CAD build for the part. Positions are in the model's coordinates, mm. Face numbers are marked on the shaded views. Round coordinates to 2 decimals unless told otherwise and drop trailing zeros. Order: outer loops, then holes, each group sorted by start corner. A loop starts at its lowest first (then second) coordinate and runs counter-clockwise, first axis right, second up. Notation, with made-up numbers: (41.25, 49.5) - (85.25, 49.5) arc R27 ccw to (85.25, 78.5) - close; hole circle Ø2 at (25, 11.5). An arc over 180 degrees is marked (long way). Use one line per item in the form item = value. Start each with the question number.
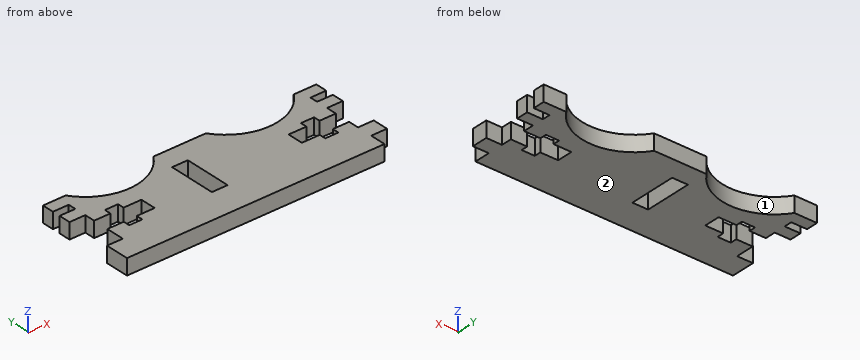
from build123d import *

# Parameters (mm, degrees)
ESBO_O1_W                     = 46
ESBO_O1_H                     = 19
RESSALTO_EXTRUS_O1_DEPTH      = 1.5
ESBO_O21_W                    = 9
ESBO_O21_H                    = 3
ESBO_O21_W_2                  = 2.5
ESBO_O21_H_2                  = 5.5
CORTE_EXTRUS_O11_DEPTH        = 3
RESSALTO_EXTRUS_O2_DEPTH      = 1.5
RESSALTO_EXTRUS_O2_DEPTH_BACK = 1.5
ESBO_O3_W                     = 3
ESBO_O3_H                     = 4.5
ESBO_O5_W                     = 3
ESBO_O5_H                     = 2.25
RESSALTO_EXTRUS_O3_DEPTH      = 1.5
RESSALTO_EXTRUS_O4_DEPTH      = 1.5
RESSALTO_EXTRUS_O4_DEPTH_BACK = 1.5
ESBO_O6_W                     = 3
ESBO_O6_H                     = 3
CORTE_EXTRUS_O2_DEPTH         = 28.721832551
CORTE_EXTRUS_O2_DEPTH_BACK    = 28.721832551
CORTE_EXTRUS_O3_DEPTH         = 28.721832551
CORTE_EXTRUS_O3_DEPTH_BACK    = 28.721832551
ESBO_O8_W                     = 3
ESBO_O8_H                     = 9


with BuildPart() as part:
    # Esboço1 → Ressalto-extrusão1 (new, symmetric)
    with BuildSketch(Plane.XY):
        Rectangle(ESBO_O1_W, ESBO_O1_H)
    extrude(amount=RESSALTO_EXTRUS_O1_DEPTH, both=True)

    # Esboço21 → Corte-extrusão11 (cut)
    with BuildSketch(Plane(origin=(-7.10842072, -2.477277924, -1.5), x_dir=(-1, 0, 0), z_dir=(0, 0, -1))):
        with Locations((-25.60842072, 2.477277924)):
            Rectangle(ESBO_O21_W, ESBO_O21_H)
        with Locations((-25.75842072, 2.477277924)):
            Rectangle(ESBO_O21_W_2, ESBO_O21_H_2)
    corte_extrus_o11 = extrude(amount=-CORTE_EXTRUS_O11_DEPTH, mode=Mode.SUBTRACT)

    # Espelhar4: Corte-extrusão11 across plane
    add(corte_extrus_o11.mirror(Plane(origin=(0, 0, 0), x_dir=(0, 0, 1), z_dir=(1, 0, 0))), mode=Mode.SUBTRACT)

    # Esboço3 → Ressalto-extrusão2 (add, two sides: drawn at the far end of the back side and taken through both)
    with BuildSketch(Plane.XY.offset(-RESSALTO_EXTRUS_O2_DEPTH_BACK)):
        with Locations((-24.5, -7.25)):
            Rectangle(ESBO_O3_W, ESBO_O3_H)
    extrude(amount=RESSALTO_EXTRUS_O2_DEPTH + RESSALTO_EXTRUS_O2_DEPTH_BACK)

    # Esboço5 → Ressalto-extrusão3 (add, symmetric)
    with BuildSketch(Plane.XY):
        with Locations((-24.5, 8.375)):
            Rectangle(ESBO_O5_W, ESBO_O5_H)
        with Locations((-24.5, 4.625)):
            Rectangle(ESBO_O5_W, ESBO_O5_H)
    ressalto_extrus_o3 = extrude(amount=RESSALTO_EXTRUS_O3_DEPTH, both=True)

    # Espelhar3: Ressalto-extrusão3 across plane
    add(ressalto_extrus_o3.mirror(Plane(origin=(0, 0, 0), x_dir=(0, 0, 1), z_dir=(1, 0, 0))))

    # Esboço6 → Ressalto-extrusão4 (add, two sides: drawn at the far end of the back side and taken through both)
    with BuildSketch(Plane.XY.offset(-RESSALTO_EXTRUS_O4_DEPTH_BACK)):
        with Locations((24.5, -5)):
            Rectangle(ESBO_O6_W, ESBO_O6_H)
    extrude(amount=RESSALTO_EXTRUS_O4_DEPTH + RESSALTO_EXTRUS_O4_DEPTH_BACK)

    # Esboço7 → Corte-extrusão2 (cut, two sides: drawn at the far end of the back side and taken through both)
    with BuildSketch(Plane.XY.offset(-CORTE_EXTRUS_O2_DEPTH_BACK)):
        with BuildLine():
            Line((-21.7, 9.5), (-4.996706912, 9.5))
            ThreePointArc((-4.996706912, 9.5), (-13.348353456, 5), (-21.7, 9.5))
        make_face()
        with BuildLine():
            Line((4.996706912, 9.5), (21.7, 9.5))
            ThreePointArc((21.7, 9.5), (13.348353456, 5), (4.996706912, 9.5))
        make_face()
    extrude(amount=CORTE_EXTRUS_O2_DEPTH + CORTE_EXTRUS_O2_DEPTH_BACK, mode=Mode.SUBTRACT)

    # Esboço8 → Corte-extrusão3 (cut, two sides: drawn at the far end of the back side and taken through both)
    with BuildSketch(Plane.XY.offset(-CORTE_EXTRUS_O3_DEPTH_BACK)):
        with Locations((-3.3, 1)):
            Rectangle(ESBO_O8_W, ESBO_O8_H)
    extrude(amount=CORTE_EXTRUS_O3_DEPTH + CORTE_EXTRUS_O3_DEPTH_BACK, mode=Mode.SUBTRACT)


solid = part.part
(1) Wall check: line 1 (X direction, y = -3, z = 0.2); line 2 (X direction, y = 2, z = 0.1); line 3 (Y direction, x = -3, z = -0.45). Give the ranges that are in metal, low to high. Write a range as [from, to].
(2) Slice it at C-C (y = -2.25). Give the cut face in (x, z).
(3) Slice it at B-B (x = 14.5). Give the cut face in (y, z), and give its area (3 significant figures).
(4) Mould opens along X. For the marked faces 1 and 2 say: pulls with the +X half, pulls with the -X half, needs draft (parallel to the pull), parting line crosses it, or undercut.
(5) Slice it at D-D (y = 8.5). Give the cut face in (x, z), and give its area (3 significant figures).
(6) Flat gauge pins, fed straight in: P1, Ø1, axis at y = 2, z = 1, coming from the -X side; P2, Ø0.6, axis at y = 2.5, z = 0.5, coming from the +X side. Where does each tip first touch, or does it go through?
(7) Slice it at A-A (y = 1). Give the cut face in (x, z).
Results list:
q1.line_1 = [-23, -4.8], [-1.8, 23]
q1.line_2 = [-23, -19.9], [-17.4, -4.8], [-1.8, 17.4], [19.9, 23]
q1.line_3 = [-9.5, -3.5], [5.5, 9.5]
q2.outline = (-23, -1.5) - (-19.9, -1.5) - (-19.9, 1.5) - (-23, 1.5) - close; (-17.4, -1.5) - (-4.8, -1.5) - (-4.8, 1.5) - (-17.4, 1.5) - close; (-1.8, -1.5) - (17.4, -1.5) - (17.4, 1.5) - (-1.8, 1.5) - close; (19.9, -1.5) - (23, -1.5) - (23, 1.5) - (19.9, 1.5) - close
q3.outline = (-9.5, -1.5) - (-1.5, -1.5) - (-1.5, 1.5) - (-9.5, 1.5) - close; (1.5, -1.5) - (5.07, -1.5) - (5.07, 1.5) - (1.5, 1.5) - close
q3.area = 34.7 mm²
q4.face_1 = undercut
q4.face_2 = needs draft
q5.outline = (-26, -1.5) - (-20.95, -1.5) - (-20.95, 1.5) - (-26, 1.5) - close; (-5.75, -1.5) - (5.75, -1.5) - (5.75, 1.5) - (-5.75, 1.5) - close; (20.95, -1.5) - (26, -1.5) - (26, 1.5) - (20.95, 1.5) - close
q5.area = 64.8 mm²
q6.P1 = -23
q6.P2 = 23
q7.outline = (-14, -1.5) - (-4.8, -1.5) - (-4.8, 1.5) - (-14, 1.5) - close; (-1.8, -1.5) - (14, -1.5) - (14, 1.5) - (-1.8, 1.5) - close
